Here's the drawing with two shaded views (mm, measured from the low corner). I have some questions. Round coordinates to 2 decimals unless told otherwise and drop trailing zeros. Use one line per item in the form item = value.
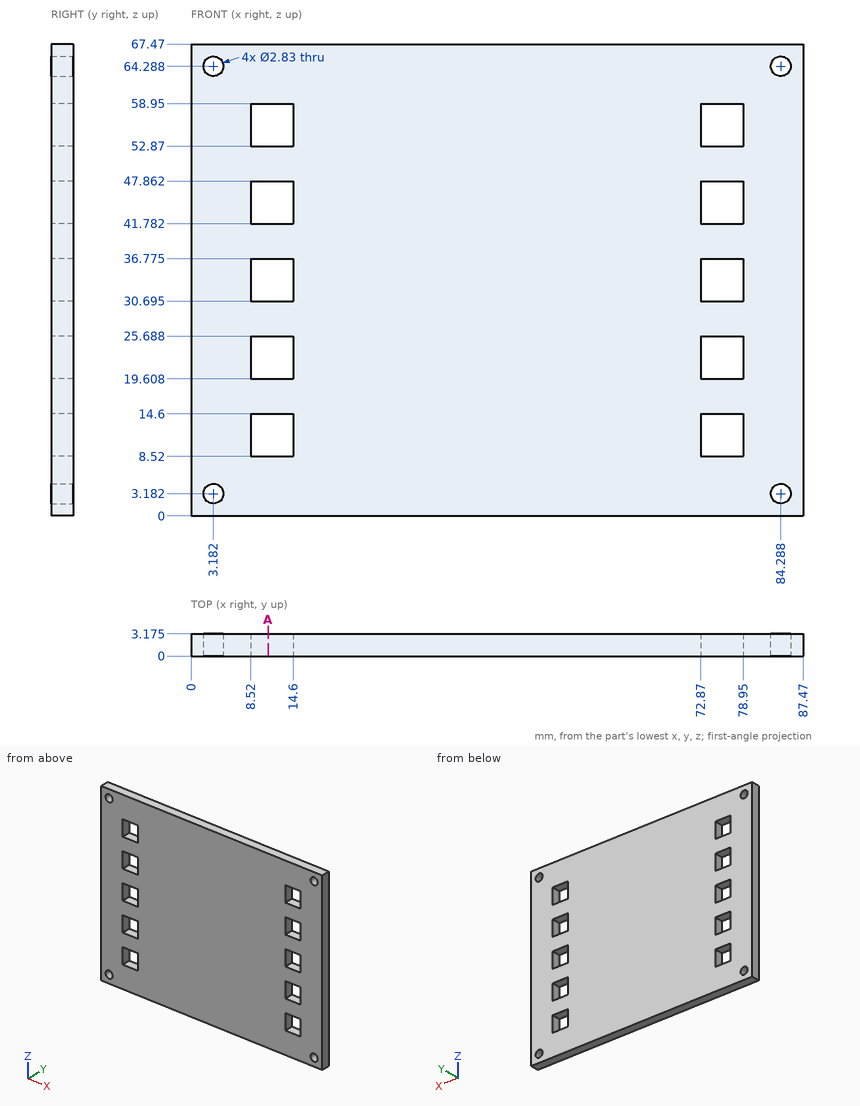
1. For P1, Ø3.5, axis at x = 84.29, z = 3.18, coming from the +Y side (1 decimal), with a flat end and sliding along its axis, tell me the tip position at first contact or that it passes through.
Solution:
P1 = 3.2
2. If we section it at A-A, the plane x = 11: Count the separate pieces of the cut face and the enclosed holes in it, plus the area to 3 significant figures.
Solution:
separate_pieces = 6
enclosed_holes = 0
area = 118 mm^2
3. Please list where these lines run through material, in increasing order: line 1 along X through (y, z) = (3, 43); line 2 along Z through (x, y) = (4, 3.05) (1 decimal).
Solution:
line_1 = 0 to 8.52, 14.6 to 72.87, 78.95 to 87.47
line_2 = 0 to 2, 4.3 to 63.1, 65.4 to 67.5
